Build history of the part. All positions in model axes, mm. Face numbers are marked on the shaded views. A direction names the side the tool comes from. Round coordinates to 2 decimals unless told otherwise and drop trailing zeros. Write each loop counter-clockwise with the first axis right and the second up, starting at its lowest first coordinate (ties: lowest second). Pieces come first, ordered by that corner, then holes. Notation, with made-up numbers: (32, 74.5) - (78, 74.5) arc R33 cw to (78, 102.5) - close; hole circle Ø5 at (-40, 69). An arc over 180 degrees is marked (long way). Write each question's results on one line, items separated by ' | '.
from build123d import *

# Parameters (mm, degrees)
SKETCH_1_W          = 272
SKETCH_1_H          = 140
EXTRUDE_1_DEPTH     = 140
SKETCH_2_W          = 252
SKETCH_2_H          = 100
CUT_EXTRUDE_1_DEPTH = 110
SKETCH_8_W          = 12
SKETCH_8_H          = 12
EXTRUDE_2_DEPTH     = 10
SKETCH_9_R          = 14.49
SKETCH_9_R_2        = 4.49
EXTRUDE_1_2_DEPTH   = 12
SKETCH_11_R         = 4.49
CUT_EXTRUDE_5_DEPTH = 298.354040116
SKETCH_13_W         = 150
SKETCH_13_H         = 140
CUT_EXTRUDE_7_DEPTH = 239.346904019
SKETCH_14_W         = 98.139384751
SKETCH_14_H         = 13
EXTRUDE_3_DEPTH     = 50
SKETCH_15_R         = 3
CUT_EXTRUDE_8_DEPTH = 231.670688982


with BuildPart() as part:
    # 草圖1 → Extrude 1 (new body)
    with BuildSketch(Plane(origin=(0, 0, 0), x_dir=(1, 0, 0), z_dir=(0, 1, 0))):
        with Locations((26.536585366, -7.390243902)):
            Rectangle(SKETCH_1_W, SKETCH_1_H)
    extrude(amount=EXTRUDE_1_DEPTH)

    # 草圖2 → 除料-伸長1 (cut)
    with BuildSketch(Plane(origin=(0, 140, 0), x_dir=(1, 0, 0), z_dir=(0, 1, 0))):
        with Locations((16.536585366, -7.390243902)):
            Rectangle(SKETCH_2_W, SKETCH_2_H)
    extrude(amount=-CUT_EXTRUDE_1_DEPTH, mode=Mode.SUBTRACT)

    # 草圖8 → 填料-伸長2 (add)
    with BuildSketch(Plane.XY.offset(77.390243902)):
        with Locations((121.536585366, 126)):
            Rectangle(SKETCH_8_W, SKETCH_8_H)
    extrude(amount=EXTRUDE_2_DEPTH)

    # 草圖9 → Extrude 1 2 (add)
    with BuildSketch(Plane(origin=(127.536585366, 0, 0), x_dir=(0, 0, -1), z_dir=(1, 0, 0))):
        with Locations((-89.390243902, 132)):
            Circle(SKETCH_9_R)
        with Locations((-89.390243902, 132)):
            Circle(SKETCH_9_R_2, mode=Mode.SUBTRACT)
    extrude(amount=-EXTRUDE_1_2_DEPTH)

    # 草圖11 → 除料-伸長5 (cut, through all)
    with BuildSketch(Plane(origin=(127.536585366, 0, 0), x_dir=(0, 0, -1), z_dir=(1, 0, 0))):
        with Locations((-89.390243902, 132)):
            Circle(SKETCH_11_R)
    extrude(amount=-CUT_EXTRUDE_5_DEPTH, mode=Mode.SUBTRACT)

    # 草圖13 → 除料-伸長7 (cut, through all)
    with BuildSketch(Plane(origin=(0, 140, 0), x_dir=(1, 0, 0), z_dir=(0, 1, 0))):
        with Locations((-34.463414634, -7.390243902)):
            Rectangle(SKETCH_13_W, SKETCH_13_H)
    extrude(amount=-CUT_EXTRUDE_7_DEPTH, mode=Mode.SUBTRACT)

    # 草圖14 → 填料-伸長3 (add)
    with BuildSketch(Plane.ZY.offset(-40.536585366)):
        with Locations((6.459936277, 13.5)):
            Rectangle(SKETCH_14_W, SKETCH_14_H)
    extrude(amount=EXTRUDE_3_DEPTH)

    # 草圖15 → 除料-伸長8 (cut, through all)
    with BuildSketch(Plane(origin=(0, 20, 0), x_dir=(1, 0, 0), z_dir=(0, 1, 0))):
        with Locations(Location((10.536585366, -7.390243902, 0), (0, 0, 270))):
            Circle(SKETCH_15_R)
    extrude(amount=-CUT_EXTRUDE_8_DEPTH, mode=Mode.SUBTRACT)


solid = part.part
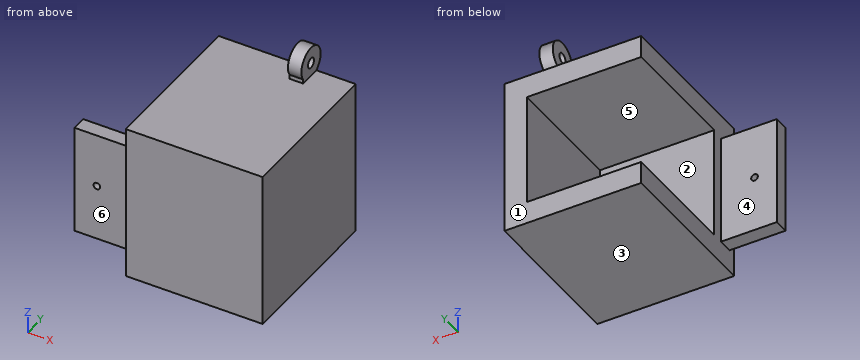
(1) Slice it at D-D, the plane z = -29. Write the cut outline in (x, y), and give its area (3 significant figures).
Worked answers:
outline: (-9.46, 7) - (40.54, 7) - (40.54, 0) - (162.54, 0) - (162.54, 140) - (142.54, 140) - (142.54, 30) - (40.54, 30) - (40.54, 20) - (-9.46, 20) - close | area: 6,510 mm2
(2) Tool access for the marked faces 4, 5 and 6: list every direction of +Z, -Z, +X, -X, +Y, -Y with a clear straight run to the whole face (end or side of a thin tool).
Worked answers:
face 4: +Z, -Z, -X, +Y | face 5: -X, +Y | face 6: +Z, -Z, -X, -Y
(3) Two-plate mould, pull along Z, no slides. Class the marked faces 1, 2 and 3: released by +Z, released by -Z, zero draft, split by the parting line, or undercut.
Worked answers:
face 1: zero draft | face 2: undercut | face 3: released by -Z
(4) Slice it at B-B, the plane x = 121. Write the cut outline in (y, z).
Worked answers:
outline: (0, -62.61) - (140, -62.61) - (140, -42.61) - (30, -42.61) - (30, 57.39) - (140, 57.39) - (140, 77.31) arc R14.49 ccw (long way) to (120, 81.27) - (120, 77.39) - (0, 77.39) - close; hole circle Ø8.98 at (132, 89.39)
(5) Slice it at C-C, the plane y = 54.5. Write the cut outline in (x, z).
Worked answers:
outline: (40.54, -62.61) - (162.54, -62.61) - (162.54, 77.39) - (40.54, 77.39) - (40.54, 57.39) - (142.54, 57.39) - (142.54, -42.61) - (40.54, -42.61) - close
(6) Drill centre lines: probe 1 along Z at (x, y) = (43, 113); probe 2 along Y at (x, z) = (141, -5.5); probe 3 along X at (y, z) = (89, 20.5). Where is each one in solid material? Low to high. Write a range as [from, to].
Worked answers:
probe 1: z = [-62.61, -42.61], [57.39, 77.39] | probe 2: y = [0, 30] | probe 3: x = [142.54, 162.54]
(7) Flat gauge pins, fed straight in: pin 1 Ø8 at (x, y) = (112, 82) entering from +Z; pin 2 Ø4 at (x, z) = (85.5, 78) entering from -Y; pin 3 Ø2 at (x, z) = (55.5, -16) entering from +Y; pin 4 Ø1.9 at (x, z) = (119.5, 78.5) entering from -Y. Where does each tip first touch, or does it go through?
Worked answers:
pin 1: stops at z = 77.39 | pin 2: stops at y = 0 | pin 3: stops at y = 30 | pin 4: stops at y = 120
(8) Slice it at A-A, the plane y = 132. Write the cut outline in (x, z), and give its area (3 significant figures).
Worked answers:
outline: (40.54, -62.61) - (162.54, -62.61) - (162.54, 77.39) - (127.54, 77.39) - (127.54, 84.9) - (115.54, 84.9) - (115.54, 77.39) - (40.54, 77.39) - (40.54, 57.39) - (142.54, 57.39) - (142.54, -42.61) - (40.54, -42.61) - close; (115.54, 93.88) - (127.54, 93.88) - (127.54, 103.88) - (115.54, 103.88) - close | area: 7,090 mm2
